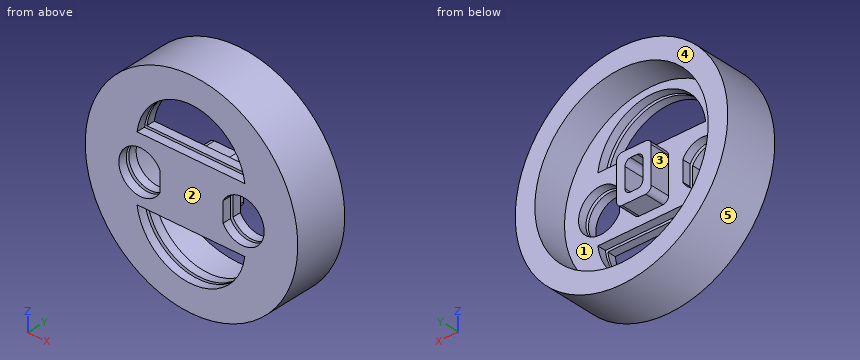
from build123d import *

# Parameters (mm, degrees)
SKETCH4_R           = 17
BOSS_EXTRUDE3_DEPTH = 6
SHELL4_T            = 0.5
SKETCH5_W           = 3.2
SKETCH5_H           = 5.5
BOSS_EXTRUDE4_DEPTH = 5
SHELL5_T            = 1.5
CUT_EXTRUDE2_DEPTH  = 69.741433184
FILLET1_R           = 1


with BuildPart() as part:
    # Sketch4 → Boss-Extrude3 (new body)
    with BuildSketch(Plane(origin=(0, 0, 0), x_dir=(1, 0, 0), z_dir=(0, 1, 0))):
        with Locations(Location((0, -46.79046007, 0), (0, 0, 270))):
            Circle(SKETCH4_R)
    extrude(amount=BOSS_EXTRUDE3_DEPTH)

    # Shell4
    shell4_openings = [part.faces().sort_by_distance(p)[0] for p in [
        (0, 6, 46.79046007),
    ]]
    offset(amount=SHELL4_T, openings=shell4_openings, kind=Kind.INTERSECTION)

    # Sketch5 → Boss-Extrude4 (add)
    with BuildSketch(Plane(origin=(0, 0, 0), x_dir=(1, 0, 0), z_dir=(0, 1, 0))):
        with Locations((0, -46.79046007)):
            Rectangle(SKETCH5_W, SKETCH5_H)
    extrude(amount=BOSS_EXTRUDE4_DEPTH)

    # Shell5
    shell5_openings = [part.faces().sort_by_distance(p)[0] for p in [
        (0, 5, 46.79046007),
    ]]
    offset(amount=SHELL5_T, openings=shell5_openings, kind=Kind.INTERSECTION)

    # Sketch8 → Cut-Extrude2 (cut, through all)
    with BuildSketch(Plane(origin=(0, 1.5, 0), x_dir=(1, 0, 0), z_dir=(0, 1, 0))):
        with BuildLine():
            Line((-9.736425903, -40.96944233), (9.535773011, -40.96944233))
            ThreePointArc((9.535773011, -40.96944233), (-0.100326446, -32.500466178), (-9.736425903, -40.96944233))
        make_face()
        with BuildLine():
            Line((-9.736425903, -52.61147781), (9.535773011, -52.61147781))
            ThreePointArc((9.535773011, -52.61147781), (-0.100326446, -61.080453963), (-9.736425903, -52.61147781))
        make_face()
        with BuildLine():
            Line((-5.651322976, -44.628261801), (-5.651322976, -48.229929487))
            ThreePointArc((-5.651322976, -48.229929487), (-12.990843168, -46.429095644), (-5.651322976, -44.628261801))
        make_face()
        with BuildLine():
            Line((5.651322976, -44.628261801), (5.651322976, -48.229929487))
            ThreePointArc((5.651322976, -48.229929487), (12.990843168, -46.429095644), (5.651322976, -44.628261801))
        make_face()
    extrude(amount=-CUT_EXTRUDE2_DEPTH, mode=Mode.SUBTRACT)

    # Fillet1
    fillet1_edges = [part.edges().sort_by_distance(p)[0] for p in [
        (3.1, 3.25, 51.04046007),
        (3.1, 3.25, 42.54046007),
        (-3.1, 3.25, 42.54046007),
        (-3.1, 3.25, 51.04046007),
        (1.6, 2.5, 49.54046007),
        (1.6, 2.5, 44.04046007),
        (-1.6, 2.5, 44.04046007),
        (-1.6, 2.5, 49.54046007),
    ]]
    fillet(fillet1_edges, radius=FILLET1_R)


solid = part.part
Can you work these out from the model? Positions are in its coordinate system, mm. Face numbers are marked on the shaded views. A direction names the side the tool comes from. Coordinates: 2 decimals unless noted, no trailing zeros. Write each loop counter-clockwise with the first axis right and the second up, starting at its lowest first coordinate (ties: lowest second). Pieces come first, ordered by that corner, then holes. Notation, with made-up numbers: (57.25, 75.25) - (88.25, 75.25) arc R32 cw to (88.25, 104.25) - close; hole circle Ø6 at (7, 69). An arc over 180 degrees is marked (long way). Return JSON: item names as keys, results as strings. Group by question number.
Item 1: Which directions (+Z, -Z, +X, -X, +Y, -Y) give clear straight access to the entire face, cutting with the end or side of a thin tool? Please do the marked faces 1 and 2.
Item 2: We'd pull the mould along Z, two halves only. Please class the marked faces 3, 4 and 5: pulls with the +Z half, pulls with the -Z half, needs draft (parallel to the pull), parting line crosses it, or undercut.
Item 3: Please list where these lines run through material, in increasing order: probe 1 along Z at (x, y) = (5, -0.75); probe 2 along X at (y, z) = (4, 60.5); probe 3 along X at (y, z) = (2.25, 38).
Item 4: If we section it at B-B (z = 34): Write out the boundary of the cut face in (x, y).
Item 5: If we section it at D-D (z = 59): Write out the boundary of the cut face in (x, y).
Item 6: I'm going to push flat-ended pins straight in: pin 1 Ø2 at (x, y) = (9, 1.5) entering from +Z; pin 2 Ø7 at (x, z) = (-9.1, 46.43) entering from +Y; pin 3 Ø15.5 at (x, z) = (-7.5, 47.5) entering from +Y; pin 4 Ø12 at (x, z) = (-6, 55) entering from +Y. Where does each tip first touch, or does it pass through?
Item 7: If we section it at C-C (x = 0): Count the separate pieces of the cut face and the enclosed holes in it, then the cut area to 3 significant figures.
Item 8: If we section it at A-A (y = 0.75): Write out the boundary of the cut face in (x, z).
Return value:
{
 "1": {"face 1": "+Y", "face 2": "+Z, -Z, +X, -X, -Y"},
 "2": {"face 3": "undercut", "face 4": "needs draft", "face 5": "parting line crosses it"},
 "3": {"probe 1": "z = 28.46 to 33.95, 40.97 to 52.61, 59.63 to 65.12", "probe 2": "x = -13.15 to -10.88, -10.05 to -7.23, 7.23 to 10.05, 10.88 to 13.15", "probe 3": "x = -16.84 to -15.13, -14.55 to -12.77, 12.77 to 14.55, 15.13 to 16.84"},
 "4": {"outline": "(-14.05, -2) - (-5.29, -2) - (-5.29, -0.5) - (-11.94, -0.5) - (-11.94, 6) - (-11.2, 6) - (-11.2, 0) - (-5.29, 0) - (-5.29, 1.5) - (-8.76, 1.5) - (-8.76, 7.5) - (-14.05, 7.5) - close; (5.09, -2) - (14.05, -2) - (14.05, 7.5) - (8.76, 7.5) - (8.76, 1.5) - (5.09, 1.5) - (5.09, 0) - (11.2, 0) - (11.2, 6) - (11.94, 6) - (11.94, -0.5) - (5.09, -0.5) - close"},
 "5": {"outline": "(-14.56, -2) - (-6.11, -2) - (-6.11, -0.5) - (-12.54, -0.5) - (-12.54, 6) - (-11.83, 6) - (-11.83, 0) - (-6.11, 0) - (-6.11, 1.5) - (-9.55, 1.5) - (-9.55, 7.5) - (-14.56, 7.5) - close; (5.91, -2) - (14.56, -2) - (14.56, 7.5) - (9.55, 7.5) - (9.55, 1.5) - (5.91, 1.5) - (5.91, 0) - (11.83, 0) - (11.83, 6) - (12.54, 6) - (12.54, -0.5) - (5.91, -0.5) - close"},
 "6": {"pin 1": "stops at z = 64.02", "pin 2": "stops at y = 1.5", "pin 3": "stops at y = 5", "pin 4": "stops at y = 7.5"},
 "7": {"separate pieces": "5", "enclosed holes": "0", "area": "103 mm^2"},
 "8": {"outline": "circle Ø38 at (0, 46.79); circle Ø34 at (0, 46.79); hole circle Ø35 at (0, 46.79); hole (-9.74, 40.97) arc R9.72 ccw to (9.54, 40.97) - close; hole (-9.74, 52.61) - (9.54, 52.61) arc R9.72 ccw to start; hole (-5.65, 44.63) - (-5.65, 48.23) arc R3.89 ccw (long way) to start; hole (-1.6, 45.04) arc R1 ccw to (-0.6, 44.04) - (0.6, 44.04) arc R1 ccw to (1.6, 45.04) - (1.6, 48.54) arc R1 ccw to (0.6, 49.54) - (-0.6, 49.54) arc R1 ccw to (-1.6, 48.54) - close; hole (5.65, 44.63) arc R3.89 ccw (long way) to (5.65, 48.23) - close"}
}
